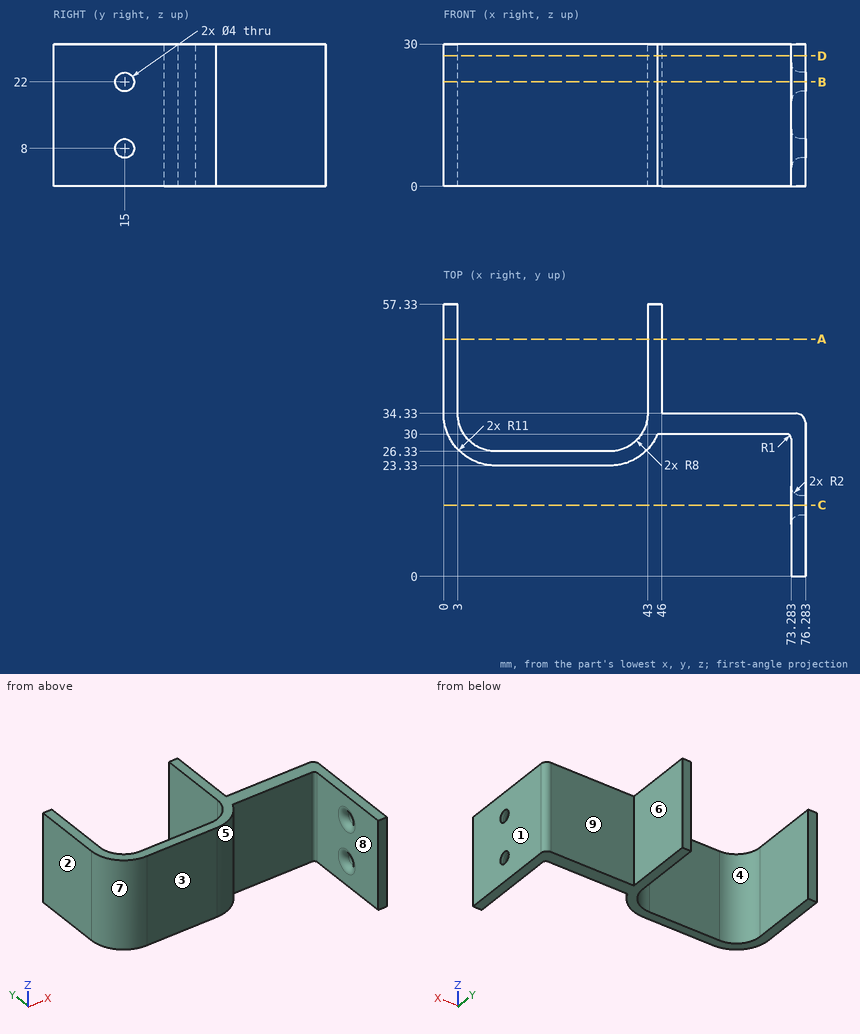
Job drawing, mm, ordinate dimensions from the low corner. One solid piece. A direction names the side the tool comes from. Coordinates: 2 decimals unless noted, no trailing zeros. Loops run counter-clockwise (first coordinate to the right, second up) from the corner with the lowest first, then second, coordinate; pieces in that order, holes last. Notation, with made-up numbers: (67, 39.25) - (94, 39.25) arc R36 ccw to (94, 75.25) - close; hole circle Ø9 at (-40, -6.5). An arc over 180 degrees is marked (long way). Write item = value, one per line. Start each with the question number.
Q1. Cut at D-D, the plane z = 27.5. List the corners of the cut face in (x, y).
Q2. Which spindle directions (+Z, -Z, +X, -X, +Y, -Y) get a long thin tool onto all of the face, cutting with end or side? Do the marked faces 1, 2, 3, 4 and 5. Say none if no direction does.
Q3. Cut at A-A, the plane y = 50. List the corners of the cut face in (x, z).
Q4. Cut at B-B, the plane z = 22. List the corners of the cut face in (x, y).
Q5. Cut at C-C, the plane y = 15. List the corners of the cut face in (x, z).
Q6. Pull direction X, two halves, no side cores. Call the marked faces 6, 7, 8 and 9: pulls with the +X half, pulls with the -X half, needs draft (parallel to the pull), parting line crosses it, or undercut.
Q7. Flat gauge pins, fed straight in: pin 1 Ø4 at (y, z) = (6, 26) entering from -X; pin 2 Ø3 at (y, z) = (49.5, 13) entering from +X; pin 3 Ø3 at (x, z) = (36, 25.5) entering from -Y; pin 4 Ø3.5 at (y, z) = (15, 8) entering from -X. Where does each tip first touch, or does it go through?
Q8. Drill centre lines: L1, parallel to Z at x = 75, y = 15; L2, parallel to X at y = 35.5, z = 9.5; L3, parallel to X at y = 28, z = 15 (1 decimal). Where is each one in solid material? Low to high.
Computed:
q1.outline = (0, 34.33) arc R11 ccw to (11, 23.33) - (35, 23.33) arc R11 ccw to (45.11, 30) - (72.28, 30) arc R1 cw to (73.28, 29) - (73.28, 0) - (76.28, 0) - (76.28, 32.33) arc R2 ccw to (74.28, 34.33) - (46, 34.33) - (46, 57.33) - (43, 57.33) - (43, 34.33) arc R8 cw to (35, 26.33) - (11, 26.33) arc R8 cw to (3, 34.33) - (3, 57.33) - (0, 57.33) - close
q2.face_1 = +Z, -Z, +X, +Y, -Y
q2.face_2 = +Z, -Z, -X, +Y, -Y
q2.face_3 = +Z, -Z, -X, -Y
q2.face_4 = +Z, -Z, +Y
q2.face_5 = +Z, -Z, -Y
q3.outline = (0, 0) - (3, 0) - (3, 30) - (0, 30) - close; (43, 0) - (46, 0) - (46, 30) - (43, 30) - close
q4.outline = (0, 34.33) arc R11 ccw to (11, 23.33) - (35, 23.33) arc R11 ccw to (45.11, 30) - (72.28, 30) arc R1 cw to (73.28, 29) - (73.28, 19) arc R2 ccw to (75.28, 17) - (76.28, 17) - (76.28, 32.33) arc R2 ccw to (74.28, 34.33) - (46, 34.33) - (46, 57.33) - (43, 57.33) - (43, 34.33) arc R8 cw to (35, 26.33) - (11, 26.33) arc R8 cw to (3, 34.33) - (3, 57.33) - (0, 57.33) - close; (73.28, 0) - (76.28, 0) - (76.28, 13) - (75.28, 13) arc R2 ccw to (73.28, 11) - close
q5.outline = (73.28, 0) - (76.28, 0) - (76.28, 6) - (75.28, 6) arc R2 ccw to (73.28, 4) - close; (73.28, 12) arc R2 ccw to (75.28, 10) - (76.28, 10) - (76.28, 20) - (75.28, 20) arc R2 ccw to (73.28, 18) - close; (73.28, 26) arc R2 ccw to (75.28, 24) - (76.28, 24) - (76.28, 30) - (73.28, 30) - close
q6.face_6 = pulls with the +X half
q6.face_7 = pulls with the -X half
q6.face_8 = undercut
q6.face_9 = needs draft
q7.pin_1 = 73.28
q7.pin_2 = 46
q7.pin_3 = 23.33
q7.pin_4 = through
q8.L1 = 0 to 5.98, 10.02 to 19.98, 24.02 to 30
q8.L2 = 0 to 3, 43 to 46
q8.L3 = 2 to 6.1, 39.9 to 44, 73.3 to 76.3
